Model file for the job. Use its own axes, mm. Face numbers are marked on the shaded views. A direction names the side the tool comes from. Round coordinates to 2 decimals unless told otherwise and drop trailing zeros. Loops run counter-clockwise (first coordinate to the right, second up) from the corner with the lowest first, then second, coordinate; pieces in that order, holes last. Notation, with made-up numbers: (5.5, 38) - (40.5, 38) arc R21 cw to (40.5, 45) - close; hole circle Ø7 at (28, 67). An arc over 180 degrees is marked (long way). Use one line per item in the form item = value.
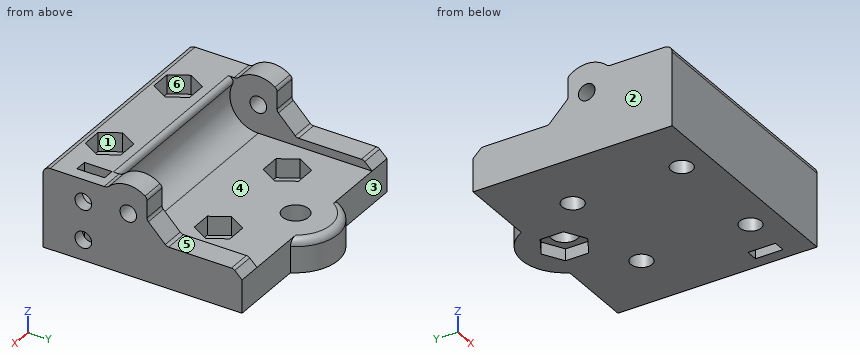
from build123d import *

# Parameters (mm, degrees)
BOSS_EXTRUDE1_DEPTH = 24.25
BOSS_EXTRUDE2_DEPTH = 7
SKETCH2_R           = 2.25
SKETCH2_R_2         = 2.75
CUT_EXTRUDE1_DEPTH  = 30
RIB2_START          = -5
RIB2_DEPTH          = 5
SKETCH11_R          = 1.75
CUT_EXTRUDE3_DEPTH  = 59.320283327
CUT_EXTRUDE5_DEPTH  = 4
CUT_EXTRUDE6_DEPTH  = 2.5
FILLET1_R           = 1
CUT_EXTRUDE7_DEPTH  = 4
FILLET2_R           = 1.5
SKETCH16_R          = 1.75
CUT_EXTRUDE8_DEPTH  = 5
CUT_EXTRUDE11_DEPTH = 2.5


# Read off the part's stored shape, not the designer's step: Rib2
with BuildPart() as part:
    # Sketch1 → Boss-Extrude1 (new, symmetric)
    with BuildSketch(Plane(origin=(0, 0, 0), x_dir=(0, 0, -1), z_dir=(1, 0, 0))):
        with BuildLine():
            Line((-2.5, 13.03872504), (4.5, 13.03872504))
            Line((4.5, 13.03872504), (4.5, -28.96127496))
            Line((4.5, -28.96127496), (-12.5, -28.96127496))
            Line((-12.5, -28.96127496), (-12.5, -15.433410915))
            ThreePointArc((-12.5, -15.433410915), (-6.050510257, -16.438500535), (-2.5, -10.96127496))
            Line((-2.5, -10.96127496), (-2.5, 13.03872504))
        make_face()
    extrude(amount=BOSS_EXTRUDE1_DEPTH, both=True)

    # Sketch8 → Boss-Extrude2 (add)
    with BuildSketch(Plane(origin=(0, 0, -4.5), x_dir=(-1, 0, 0), z_dir=(0, 0, -1))):
        with BuildLine():
            Line((-8.062257748, 13.03872504), (8.062257748, 13.03872504))
            ThreePointArc((8.062257748, 13.03872504), (0, 18.03872504), (-8.062257748, 13.03872504))
        make_face()
    extrude(amount=-BOSS_EXTRUDE2_DEPTH)

    # Sketch2 → Cut-Extrude1 (cut)
    with BuildSketch(Plane(origin=(0, 0, -4.5), x_dir=(-1, 0, 0), z_dir=(0, 0, -1))):
        with Locations(Location((11.5, 0.03872504, 0), (0, 0, 90))):
            Circle(SKETCH2_R)
        with Locations(Location((-11.5, 0.03872504, 0), (0, 0, 90))):
            Circle(SKETCH2_R)
        with Locations(Location((-11.5, -22.96127496, 0), (0, 0, 90))):
            Circle(SKETCH2_R)
        with Locations(Location((11.5, -22.96127496, 0), (0, 0, 90))):
            Circle(SKETCH2_R)
        with Locations(Location((0, 9.03872504, 0), (0, 0, 90))):
            Circle(SKETCH2_R_2)
    extrude(amount=-CUT_EXTRUDE1_DEPTH, mode=Mode.SUBTRACT)

    # Rib2 outline → Rib2 (add)
    with BuildSketch(Plane(origin=(24.25, 0, 0), x_dir=(0, 0, -1), z_dir=(1, 0, 0)).offset(RIB2_START)):
        with BuildLine():
            Line((-2.5, 13.03872504), (-4.258517887, 11.208482718))
            Line((-4.258517887, 11.208482718), (-4.258517887, -2.878129508))
            Line((-4.258517887, -2.878129508), (-8.467587637, -7.01127496))
            Line((-8.467587637, -7.01127496), (-13.016359153, -7.01127496))
            ThreePointArc((-13.016359153, -7.01127496), (-14.488755031, -11.328444107), (-12.5, -15.433410915))
            ThreePointArc((-12.5, -15.433410915), (-6.050510257, -16.438500535), (-2.5, -10.96127496))
            Line((-2.5, -10.96127496), (-2.5, 13.03872504))
        make_face()
    rib2 = extrude(amount=RIB2_DEPTH)

    # Mirror1: Rib2 across plane
    add(rib2.mirror(Plane(origin=(0, 0, 0), x_dir=(0, 0, 1), z_dir=(1, 0, 0))))

    # Sketch11 → Cut-Extrude3 (cut, through all)
    with BuildSketch(Plane(origin=(24.25, 0, 0), x_dir=(0, 0, -1), z_dir=(1, 0, 0))):
        with Locations((-8.5, -10.96127496)):
            Circle(SKETCH11_R)
    extrude(amount=-CUT_EXTRUDE3_DEPTH, mode=Mode.SUBTRACT)

    # Sketch12 → Cut-Extrude5 (cut)
    with BuildSketch(Plane(origin=(0, 0, -1.5), x_dir=(-1, 0, 0), z_dir=(0, 0, -1))):
        Polygon((15.830127019, 0.03872504), (13.665063509, 3.78872504), (9.334936491, 3.78872504), (7.169872981, 0.03872504), (9.334936491, -3.71127496), (13.665063509, -3.71127496), align=None)
        Polygon((-7.169872981, 0.03872504), (-9.334936491, 3.78872504), (-13.665063509, 3.78872504), (-15.830127019, 0.03872504), (-13.665063509, -3.71127496), (-9.334936491, -3.71127496), align=None)
    extrude(amount=-CUT_EXTRUDE5_DEPTH, mode=Mode.SUBTRACT)

    # Sketch14 → Cut-Extrude6 (cut)
    with BuildSketch(Plane(origin=(0, 0, -4.5), x_dir=(-1, 0, 0), z_dir=(0, 0, -1))):
        Polygon((0, 13.946202328), (-4.25, 11.492463684), (-4.25, 6.584986396), (0, 4.131247752), (4.25, 6.584986396), (4.25, 11.492463684), align=None)
    extrude(amount=-CUT_EXTRUDE6_DEPTH, mode=Mode.SUBTRACT)

    # Fillet1
    fillet1_edges = [part.edges().sort_by_distance(p)[0] for p in [
        (0, -15.433410915, 12.5),
        (21.75, -2.878129508, 4.258517887),
        (21.75, -7.01127496, 8.467587637),
        (21.75, -7.01127496, 13.016359153),
        (21.75, 11.208482718, 4.258517887),
        (-21.75, -7.01127496, 13.016359153),
        (-21.75, -7.01127496, 8.467587637),
        (-21.75, -2.878129508, 4.258517887),
        (-21.75, 11.208482718, 4.258517887),
    ]]
    fillet(fillet1_edges, radius=FILLET1_R)

    # Sketch15 → Cut-Extrude7 (cut)
    with BuildSketch(Plane.XY.offset(12.5)):
        Polygon((-7.169872981, -22.96127496), (-9.334936491, -19.21127496), (-13.665063509, -19.21127496), (-15.830127019, -22.96127496), (-13.665063509, -26.71127496), (-9.334936491, -26.71127496), align=None)
        Polygon((15.830127019, -22.96127496), (13.665063509, -19.21127496), (9.334936491, -19.21127496), (7.169872981, -22.96127496), (9.334936491, -26.71127496), (13.665063509, -26.71127496), align=None)
    extrude(amount=-CUT_EXTRUDE7_DEPTH, mode=Mode.SUBTRACT)

    # Fillet2
    fillet2_edges = [part.edges().sort_by_distance(p)[0] for p in [
        (0, -28.96127496, 12.5),
        (21.75, -15.433410915, 12.5),
        (0, 18.03872504, 2.5),
        (-21.75, -15.433410915, 12.5),
    ]]
    fillet(fillet2_edges, radius=FILLET2_R)

    # Sketch16 → Cut-Extrude8 (cut)
    with BuildSketch(Plane(origin=(24.25, 0, 0), x_dir=(0, 0, -1), z_dir=(1, 0, 0))):
        with Locations((0.178756589, -20.46127496)):
            Circle(SKETCH16_R)
        with Locations((-7.821243411, -20.46127496)):
            Circle(SKETCH16_R)
    extrude(amount=-CUT_EXTRUDE8_DEPTH, mode=Mode.SUBTRACT)

    # Sketch18 → Cut-Extrude11 (cut)
    with BuildSketch(Plane(origin=(19.25, 0, 0), x_dir=(0, 0, -1), z_dir=(1, 0, 0))):
        Polygon((-6.146927631, -17.56127496), (-12.752223074, -17.56127496), (-12.752223074, -23.36127496), (-6.146927631, -23.36127496), (-4.47261185, -20.46127496), align=None)
        Polygon((-1.495559192, -23.36127496), (4.713363878, -23.36127496), (4.713363878, -17.56127496), (-1.495559192, -17.56127496), (-3.169874973, -20.46127496), align=None)
    extrude(amount=CUT_EXTRUDE11_DEPTH, mode=Mode.SUBTRACT)


solid = part.part
1. Cut at B-B, the plane y = -1.5. Give the cut face in (x, z), plus the area to 3 significant figures.
Geometry check:
outline = (-24.25, -4.5) - (-13.14, -4.5) - (-13.14, -1.5) - (-14.94, -1.5) - (-14.94, 2.5) - (-19.25, 2.5) - (-19.25, 4.26) - (-24.25, 4.26) - close; (-9.86, -4.5) - (9.86, -4.5) - (9.86, -1.5) - (8.06, -1.5) - (8.06, 2.5) - (-8.06, 2.5) - (-8.06, -1.5) - (-9.86, -1.5) - close; (13.14, -4.5) - (24.25, -4.5) - (24.25, 4.26) - (19.25, 4.26) - (19.25, 2.5) - (14.94, 2.5) - (14.94, -1.5) - (13.14, -1.5) - close
area = 282 mm^2
2. Tool access for the marked faces 4, 5 and 6: list every direction of +Z, -Z, +X, -X, +Y, -Y with a clear straight run to the whole face (end or side of a thin tool).
Geometry check:
face_4 = +Z, +Y
face_5 = +Z, +X, -X, +Y
face_6 = +Z
3. Pull direction X, two halves, no side cores. Call the marked faces 1, 2 and 3: +X half, -X half, draft (parallel to the pull), parting line (faces both ways), or undercut.
Geometry check:
face_1 = undercut
face_2 = -X half
face_3 = draft
4. Cut at A-A, the plane x = 11.5. Give the cut face in (y, z), plus the area to 3 significant figures.
Geometry check:
outline = (-28.96, -4.5) - (-25.21, -4.5) - (-25.21, 8.5) - (-26.71, 8.5) - (-26.71, 12.5) - (-27.46, 12.5) arc R1.5 ccw to (-28.96, 11) - close; (-20.71, -4.5) - (-2.21, -4.5) - (-2.21, -1.5) - (-3.71, -1.5) - (-3.71, 2.5) - (-10.96, 2.5) arc R6 cw to (-16.38, 11.07) arc R1 ccw to (-17.29, 12.5) - (-19.21, 12.5) - (-19.21, 8.5) - (-20.71, 8.5) - close; (2.29, -4.5) - (13.04, -4.5) - (13.04, 2.5) - (3.79, 2.5) - (3.79, -1.5) - (2.29, -1.5) - close
area = 290 mm^2
5. Wall check: probe 1 along X at (y, z) = (2, -3); probe 2 along X at (y, z) = (-14, 8.75); probe 3 along Z at (x, y) = (2, 6.5). Give the ranges that are in metal, low to high.
Geometry check:
probe_1 = -24.25 to -12.6, -10.4 to 10.4, 12.6 to 24.25
probe_2 = -24.25 to -19.25, 19.25 to 24.25
probe_3 = -2 to 2.5
6. Cut at D-D, the plane x = 18. Give the cut face in (y, z), plus the area to 3 significant figures.
Geometry check:
outline = (-28.96, -4.5) - (13.04, -4.5) - (13.04, 2.5) - (-10.96, 2.5) arc R6 cw to (-16.38, 11.07) arc R1 ccw to (-17.29, 12.5) - (-27.46, 12.5) arc R1.5 ccw to (-28.96, 11) - close
area = 422 mm^2
7. Cut at C-C, the plane z = 0.25. Give the number of separate pieces and of enclosed holes in the cut face, plus the area to 3 significant figures.
Geometry check:
separate_pieces = 1
enclosed_holes = 5
area = 1,920 mm^2
8. Flat gauge pins, fed straight in: pin 1 (4.5 mm diameter, centred on x = 11, z = 10.5, fed in from +Y); pin 2 (2 mm diameter, centred on x = 10, z = 9, fed in from +Y); pin 3 (4 mm diameter, centred on x = 11, y = -24.5, fed in from +Z). Where does each tip first touch, or does it go through?
Geometry check:
pin_1 = -16.29
pin_2 = -16.77
pin_3 = 8.5
